Geometry check sheet. Reference: drawing and pictorial views, mm from the part's lowest x, y, z. Coordinates: 2 decimals unless noted, no trailing zeros. Write each loop counter-clockwise with the first axis right and the second up, starting at its lowest first coordinate (ties: lowest second). Pieces come first, ordered by that corner, then holes. Notation, with made-up numbers: M 85,10 L 100,10 A33 ccw 100,47 Z; hole C 10,79.5 d10. An arc over 180 degrees is marked long. One line per item, written item: value.
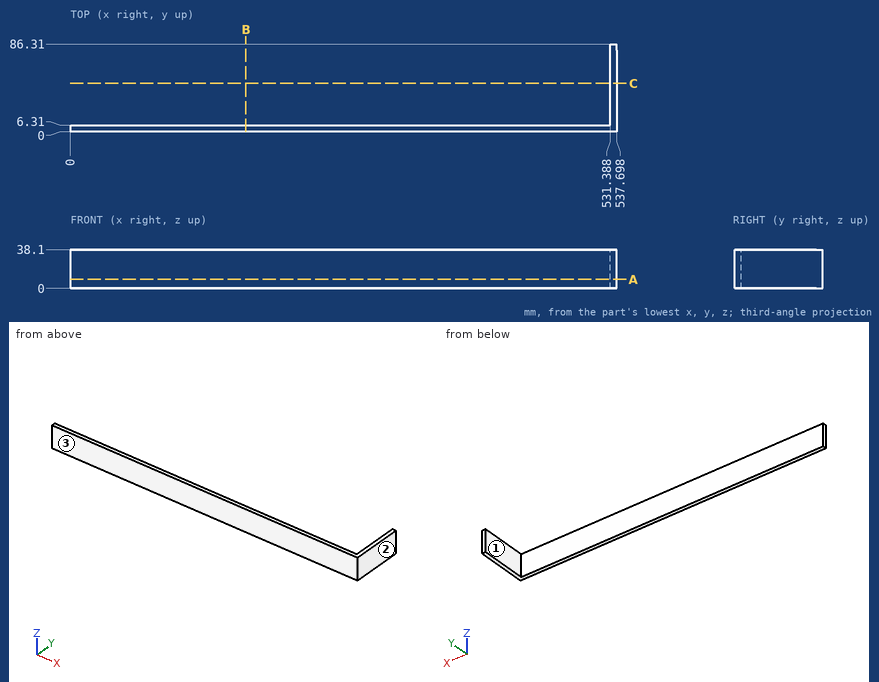
Item 1: Go/stop test with flat-tipped pins: P1, Ø12, axis at x = 80.5, z = 28.5, coming from the +Y side; P2, Ø1.5, axis at y = 23, z = 26.5, coming from the -X side. Record where each tip stops, or that it passes through.
The answers:
P1: stops at y = 6.31
P2: stops at x = 531.39
Item 2: Cross-section at A-A, the plane z = 9. Enter the section's corners in (x, y), and give its area (3 significant figures).
The answers:
outline: M 0,0 L 537.7,0 L 537.7,86.31 L 531.39,86.31 L 531.39,6.31 L 0,6.31 Z
area: 3,900 mm²
Item 3: Cross-section at C-C, the plane y = 47.5. Enter the section's corners in (x, z).
The answers:
outline: M 531.39,0 L 537.7,0 L 537.7,38.1 L 531.39,38.1 Z
Item 4: Scan lines: line 1 (X direction, y = 41, z = 4); line 2 (Y direction, x = 41.5, z = 28.5). Record each from-to range of solid material in increasing order.
The answers:
line 1: x = 531.39 to 537.7
line 2: y = 0 to 6.31
Item 5: Cross-section at B-B, the plane x = 172.5. Enter the section's corners in (y, z), and give its area (3 significant figures).
The answers:
outline: M 0,0 L 6.31,0 L 6.31,38.1 L 0,38.1 Z
area: 240 mm²
Item 6: Draft check along X on the marked faces 1, 2 and 3. Enter one of: released by +X, released by -X, zero draft, split by the parting line, or undercut.
The answers:
face 1: released by -X
face 2: released by +X
face 3: zero draft
